Check sheet for the modelled part. Datum: model origin and axes. Units: mm. Face numbers are marked on the shaded views. Round coordinates to 2 decimals unless told otherwise and drop trailing zeros. Loops run counter-clockwise (first coordinate to the right, second up) from the corner with the lowest first, then second, coordinate; pieces in that order, holes last. Notation, with made-up numbers: (9.5, 59.25) -> (59.5, 59.25) arc R18 cw to (59.5, 88.25) -> close; hole circle Ø6 at (46.25, 42). An arc over 180 degrees is marked (long way). Use one line per item in the form item = value. Start each with the question number.
(1) Sectioned sample at A-A (x = 0). Record the cut outline in (y, z), and give its area (3 significant figures).
(2) Sectioned sample at C-C (z = 2.4). Record the cut outline in (x, y), and give its area (3 significant figures).
(3) Sectioned sample at B-B (y = 0.25). Record the cut outline in (x, z).
(4) Draft check along X on the marked faces 1, 2 and 3. Enter one of: released by +X, released by -X, zero draft, split by the parting line, or undercut.
(5) Material ranges on probe 1 along Y at (x, z) = (0, 3.5); probe 2 along Z at (x, y) = (-4.25, 1.75); probe 3 along X at (y, z) = (0.25, 3.7), recorded low to high. Write a range as [from, to].
(6) Sectioned sample at D-D (y = -4.25). Record the cut outline in (x, z).
(7) Go/stop test with flat-tipped pins: pin 1 (1.5 mm diameter, centred on x = 1, z = 1, fed in from -Y); pin 2 (2 mm diameter, centred on x = 5, z = 3, fed in from -Y). Record where each tip stops, or that it passes through.
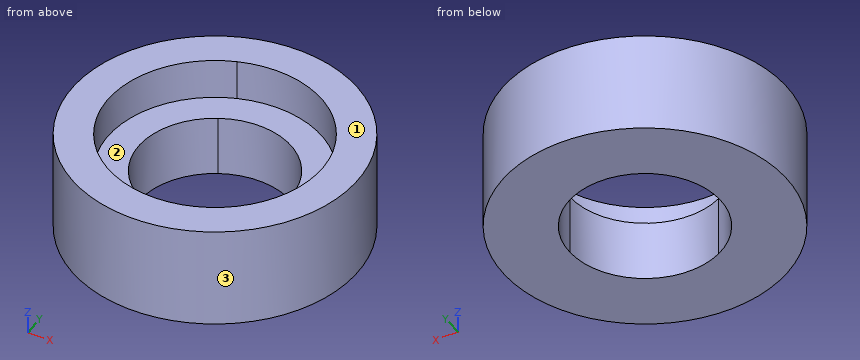
from build123d import *

# Parameters (mm, degrees)
F0_R     = 7
F1_DEPTH = 5
F2_DEPTH = 3


with BuildPart() as f1:
    # F0 (on Top) → F1 (new body)
    with BuildSketch(Plane.XY):
        Circle(F0_R)
        with BuildLine():
            ThreePointArc((-1.75, -4.9497474683), (-5.25, 0), (-1.75, 4.9497474683))
            ThreePointArc((-1.75, 4.9497474683), (3.0310889132, 4.2866070499), (5.25, 0))
            ThreePointArc((5.25, 0), (3.0310889132, -4.2866070499), (-1.75, -4.9497474683))
        make_face(mode=Mode.SUBTRACT)
    extrude(amount=F1_DEPTH)

    # F0 (on Top) → F2 (join)
    with BuildSketch(Plane.XY):
        with BuildLine():
            ThreePointArc((-1.75, 3.3166247904), (1.9364916731, 3.2113081447), (3.75, 0))
            ThreePointArc((3.75, 0), (1.9364916731, -3.2113081447), (-1.75, -3.3166247904))
            Line((-1.75, -3.3166247904), (-1.75, -4.9497474683))
            ThreePointArc((-1.75, -4.9497474683), (3.0310889132, -4.2866070499), (5.25, 0))
            ThreePointArc((5.25, 0), (3.0310889132, 4.2866070499), (-1.75, 4.9497474683))
            Line((-1.75, 4.9497474683), (-1.75, 3.3166247904))
        make_face()
        with BuildLine():
            ThreePointArc((-1.75, -3.3166247904), (-3.75, 0), (-1.75, 3.3166247904))
            Line((-1.75, 3.3166247904), (-1.75, 4.9497474683))
            ThreePointArc((-1.75, 4.9497474683), (-5.25, 0), (-1.75, -4.9497474683))
            Line((-1.75, -4.9497474683), (-1.75, -3.3166247904))
        make_face()
    extrude(amount=F2_DEPTH)


solid = f1.part
Checks:
q1.outline = (-7, 0) -> (-3.75, 0) -> (-3.75, 3) -> (-5.25, 3) -> (-5.25, 5) -> (-7, 5) -> close; (3.75, 0) -> (7, 0) -> (7, 5) -> (5.25, 5) -> (5.25, 3) -> (3.75, 3) -> close
q1.area = 26.5 mm2
q2.outline = circle Ø14 at (0, 0); hole circle Ø7.5 at (0, 0)
q2.area = 110 mm2
q3.outline = (-7, 0) -> (-3.74, 0) -> (-3.74, 3) -> (-5.24, 3) -> (-5.24, 5) -> (-7, 5) -> close; (3.74, 0) -> (7, 0) -> (7, 5) -> (5.24, 5) -> (5.24, 3) -> (3.74, 3) -> close
q4.face_1 = zero draft
q4.face_2 = undercut
q4.face_3 = split by the parting line
q5.probe_1 = [-7, -5.25], [5.25, 7]
q5.probe_2 = [0, 3]
q5.probe_3 = [-7, -5.24], [5.24, 7]
q6.outline = (-5.56, 0) -> (5.56, 0) -> (5.56, 5) -> (3.08, 5) -> (3.08, 3) -> (-3.08, 3) -> (-3.08, 5) -> (-5.56, 5) -> close
q7.pin_1 = -7
q7.pin_2 = -5.74
